from build123d import *

# Parameters (mm, degrees)
SKETCH1_W                                       = 60
SKETCH1_H                                       = 60
SKETCH1_R                                       = 2.2
SKETCH1_R_2                                     = 1.65
BOSS_EXTRUDE1_DEPTH                             = 4
CSK_FOR_M3_FLAT_HEAD_MACHINE_SCREW1_D           = 3.6
CSK_FOR_M3_FLAT_HEAD_MACHINE_SCREW1_CSINK_D     = 6.9
CSK_FOR_M3_FLAT_HEAD_MACHINE_SCREW1_CSINK_ANGLE = 90


with BuildPart() as part:
    # Sketch1 → Boss-Extrude1 (new body)
    with BuildSketch(Plane(origin=(0, 0, 0), x_dir=(1, 0, 0), z_dir=(0, 1, 0))):
        Rectangle(SKETCH1_W, SKETCH1_H)
        with Locations(Location((-25, 25, 0), (0, 0, 270))):
            Circle(SKETCH1_R, mode=Mode.SUBTRACT)
        with Locations(Location((-16, 16, 0), (0, 0, 270))):
            Circle(SKETCH1_R_2, mode=Mode.SUBTRACT)
        with Locations(Location((-25, -25, 0), (0, 0, 270))):
            Circle(SKETCH1_R, mode=Mode.SUBTRACT)
        with Locations(Location((-16, -16, 0), (0, 0, 270))):
            Circle(SKETCH1_R_2, mode=Mode.SUBTRACT)
        with Locations(Location((25, -25, 0), (0, 0, 270))):
            Circle(SKETCH1_R, mode=Mode.SUBTRACT)
        with Locations(Location((16, -16, 0), (0, 0, 270))):
            Circle(SKETCH1_R_2, mode=Mode.SUBTRACT)
        with Locations(Location((25, 25, 0), (0, 0, 270))):
            Circle(SKETCH1_R, mode=Mode.SUBTRACT)
        with Locations(Location((16, 16, 0), (0, 0, 270))):
            Circle(SKETCH1_R_2, mode=Mode.SUBTRACT)
    extrude(amount=BOSS_EXTRUDE1_DEPTH)

    # CSK for M3 Flat Head Machine Screw1 (through all)
    with Locations(Plane(origin=(16, 4, -16), x_dir=(0, 0, 1), z_dir=(0, 1, 0))):
        with Locations((0, 0), (32, 0), (32, -32), (0, -32)):
            CounterSinkHole(CSK_FOR_M3_FLAT_HEAD_MACHINE_SCREW1_D / 2, CSK_FOR_M3_FLAT_HEAD_MACHINE_SCREW1_CSINK_D / 2, counter_sink_angle=CSK_FOR_M3_FLAT_HEAD_MACHINE_SCREW1_CSINK_ANGLE)


solid = part.part
Here's how the part is built. I have some questions about the finished solid (model axes, mm). Give positions to 0.01 mm unless a question says otherwise; leave off trailing zeros. Write each loop counter-clockwise with the first axis right and the second up, starting at its lowest first coordinate (ties: lowest second). Pieces come first, ordered by that corner, then holes. Notation, with made-up numbers: (76, -12) -> (117, -12) arc R18 cw to (117, 0) -> close; hole circle Ø11 at (45, 15.5). An arc over 180 degrees is marked (long way). Use one line per item in the form item = value. Start each with the question number.
1. Imagine slicing it at B-B on x = 16. List the corners of the cut face in (y, z) for me, plus the area to 3 significant figures.
2. Thinking about a two-plate mould opening in X: for faces 1 (the face through (-27.148, 1.972, -25.477)), 2 (the face through (0, 0, 0)), 3 (the face through (-30, 2, 0)), which applies, +X half, -X half, draft (parallel to the pull), parting line (faces both ways), or undercut?
3. If I drill on L1, parallel to X at y = 1.95, z = 25; L2, parallel to X at y = 0.9, z = 16, over which ranges is the centre line in solid material (lowest first)?
4. Imagine slicing it at C-C on y = 1. State how many separate pieces and enclosed holes the cut face has, plus the area to 3 significant figures.
5. Imagine slicing it at A-A on z = 25. List the corners of the cut face in (x, y) for me, plus the area to 3 significant figures.
6. Imagine slicing it at D-D on z = -16. List the corners of the cut face in (x, y) for me, plus the area to 3 significant figures.
7. Will these pins go through, and if not, where does the flat tip stop? pin 1 Ø2.5 at (x, z) = (25, 25) entering from +Y; pin 2 Ø7 at (x, z) = (-25, 25) entering from +Y.
Entries:
q1.outline = (0, -30) -> (4, -30) -> (4, -19.45) -> (2.35, -17.8) -> (0, -17.8) -> close; (0, -14.2) -> (2.35, -14.2) -> (4, -12.55) -> (4, 12.55) -> (2.35, 14.2) -> (0, 14.2) -> close; (0, 17.8) -> (2.35, 17.8) -> (4, 19.45) -> (4, 30) -> (0, 30) -> close
q1.area = 206 mm²
q2.face_1 = undercut
q2.face_2 = draft
q2.face_3 = -X half
q3.L1 = -30 to -27.2, -22.8 to 22.8, 27.2 to 30
q3.L2 = -30 to -17.8, -14.2 to 14.2, 17.8 to 30
q4.separate_pieces = 1
q4.enclosed_holes = 8
q4.area = 3,500 mm²
q5.outline = (-30, 0) -> (-27.2, 0) -> (-27.2, 4) -> (-30, 4) -> close; (-22.8, 0) -> (22.8, 0) -> (22.8, 4) -> (-22.8, 4) -> close; (27.2, 0) -> (30, 0) -> (30, 4) -> (27.2, 4) -> close
q5.area = 205 mm²
q6.outline = (-30, 0) -> (-17.8, 0) -> (-17.8, 2.35) -> (-19.45, 4) -> (-30, 4) -> close; (-14.2, 0) -> (14.2, 0) -> (14.2, 2.35) -> (12.55, 4) -> (-12.55, 4) -> (-14.2, 2.35) -> close; (17.8, 0) -> (30, 0) -> (30, 4) -> (19.45, 4) -> (17.8, 2.35) -> close
q6.area = 206 mm²
q7.pin_1 = through
q7.pin_2 = 4
